Input: dimensioned drawing with shaded views. Units: mm. Origin: part minimum x, y, z. Round coordinates to 2 decimals unless told otherwise and drop trailing zeros. Loops run counter-clockwise (first coordinate to the right, second up) from the corner with the lowest first, then second, coordinate; pieces in that order, holes last. Notation, with made-up numbers: M 12.5,1.5 L 24.5,1.5 A22 ccw 24.5,8.5 Z; hole C 27.25,-18 d8. An arc over 180 degrees is marked long. Return JSON: item names as keys, results as strings.
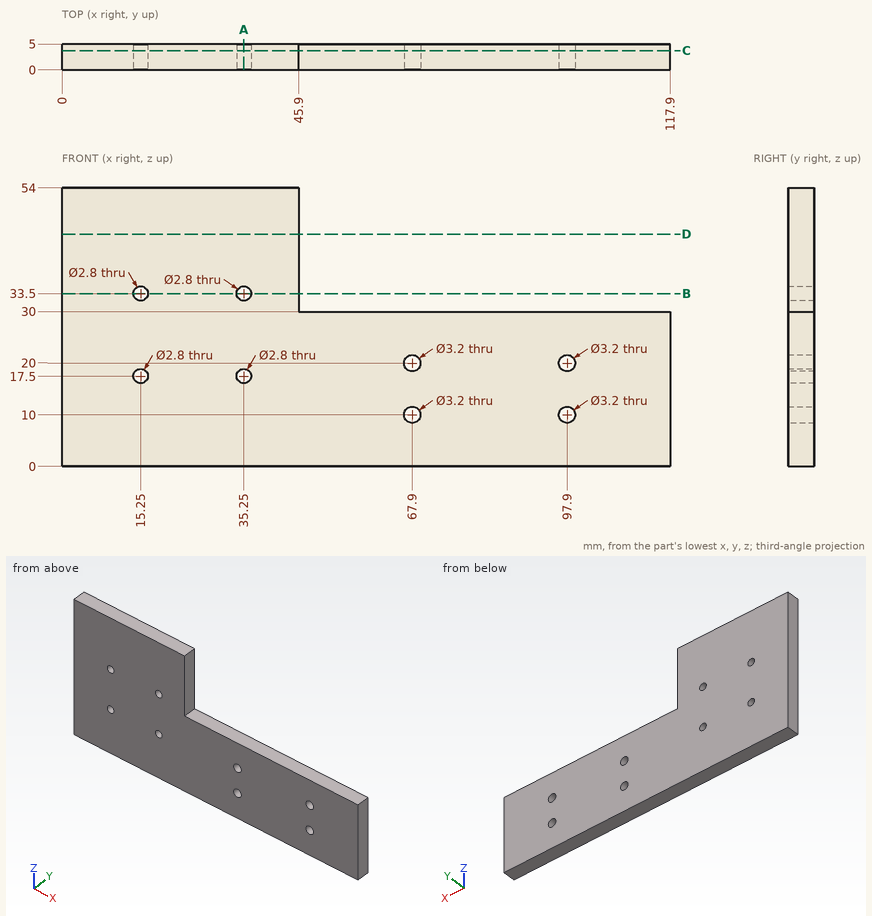
Q1. Section query D-D (z = 45). Output: boundary loops of the cut face in (x, y).
Determined:
{"outline": "M 0,0 L 45.9,0 L 45.9,5 L 0,5 Z"}
Q2. Section query B-B (z = 33.5). Output: boundary loops of the cut face in (x, y).
Determined:
{"outline": "M 0,0 L 13.85,0 L 13.85,5 L 0,5 Z; M 16.65,0 L 33.85,0 L 33.85,5 L 16.65,5 Z; M 36.65,0 L 45.9,0 L 45.9,5 L 36.65,5 Z"}
Q3. Pin query (flat end, axial travel): pin 1 (1 mm diameter, centred on x = 57, z = 19.5, fed in from -Y); pin 2 (2.5 mm diameter, centred on x = 77, y = 2.5, fed in from +Z). Return the tip coordinate at first contact, or that it passes through.
Determined:
{"pin 1": "stops at y = 0", "pin 2": "stops at z = 30"}
Q4. Material intervals for L1, parallel to X at y = 1.6, z = 20; L2, parallel to X at y = 3.8, z = 17.5; L3, parallel to Z at x = 67.9, y = 1.3, sorted ascending.
Determined:
{"L1": "x = 0 to 66.3, 69.5 to 96.3, 99.5 to 117.9", "L2": "x = 0 to 13.85, 16.65 to 33.85, 36.65 to 117.9", "L3": "z = 0 to 8.4, 11.6 to 18.4, 21.6 to 30"}
Q5. Section query A-A (x = 35.25). Output: boundary loops of the cut face in (y, z), plus the area to 3 significant figures.
Determined:
{"outline": "M 0,0 L 5,0 L 5,16.1 L 0,16.1 Z; M 0,18.9 L 5,18.9 L 5,32.1 L 0,32.1 Z; M 0,34.9 L 5,34.9 L 5,54 L 0,54 Z", "area": "242 mm^2"}
Q6. Section query C-C (y = 3.7). State how many separate pieces and enclosed holes the cut face has, plus the area to 3 significant figures.
Determined:
{"separate pieces": "1", "enclosed holes": "8", "area": "4,580 mm^2"}
